from build123d import *

# Parameters (mm, degrees)
BOSS_EXTRUDE2_DEPTH = 64
CUT_EXTRUDE3_START  = -45
CUT_EXTRUDE3_DEPTH  = 45
SKETCH7_R           = 11
CUT_EXTRUDE5_DEPTH  = 96
SKETCH8_R           = 11
CUT_EXTRUDE6_DEPTH  = 105
CUT_EXTRUDE7_START  = -45
CUT_EXTRUDE7_DEPTH  = 45
SKETCH10_W          = 13
SKETCH10_H          = 64
CUT_EXTRUDE8_DEPTH  = 45
SKETCH11_W          = 13
SKETCH11_H          = 64
CUT_EXTRUDE9_DEPTH  = 45
CUT_EXTRUDE12_DEPTH = 31
CUT_EXTRUDE13_DEPTH = 31


with BuildPart() as part:
    # Sketch1 → Boss-Extrude2 (new body)
    with BuildSketch(Plane(origin=(0, 0, 0), x_dir=(1, 0, 0), z_dir=(0, 1, 0))):
        with BuildLine():
            Line((0, -32), (114, -32))
            ThreePointArc((114, -32), (146, 0), (114, 32))
            Line((114, 32), (0, 32))
            ThreePointArc((0, 32), (-32, 0), (0, -32))
        make_face()
    extrude(amount=BOSS_EXTRUDE2_DEPTH)

    # Sketch6 → Cut-Extrude3 (cut)
    with BuildSketch(Plane(origin=(0, 64, 0), x_dir=(1, 0, 0), z_dir=(0, 1, 0)).offset(CUT_EXTRUDE3_START)):
        with BuildLine():
            Line((0, 32), (0, -32))
            ThreePointArc((0, -32), (-32, 0), (0, 32))
        make_face()
    extrude(amount=CUT_EXTRUDE3_DEPTH, mode=Mode.SUBTRACT)

    # Sketch7 → Cut-Extrude5 (cut)
    with BuildSketch(Plane(origin=(0, 64, 0), x_dir=(1, 0, 0), z_dir=(0, 1, 0))):
        with Locations(Location((0, 0, 0), (0, 0, 270))):
            Circle(SKETCH7_R)
    extrude(amount=-CUT_EXTRUDE5_DEPTH, mode=Mode.SUBTRACT)

    # Sketch8 → Cut-Extrude6 (cut)
    with BuildSketch(Plane(origin=(0, 64, 0), x_dir=(1, 0, 0), z_dir=(0, 1, 0))):
        with Locations(Location((114, 0, 0), (0, 0, 270))):
            Circle(SKETCH8_R)
    extrude(amount=-CUT_EXTRUDE6_DEPTH, mode=Mode.SUBTRACT)

    # Sketch9 → Cut-Extrude7 (cut)
    with BuildSketch(Plane(origin=(0, 64, 0), x_dir=(1, 0, 0), z_dir=(0, 1, 0)).offset(CUT_EXTRUDE7_START)):
        with BuildLine():
            Line((114, 32), (114, -32))
            ThreePointArc((114, -32), (146, 0), (114, 32))
        make_face()
    extrude(amount=CUT_EXTRUDE7_DEPTH, mode=Mode.SUBTRACT)

    # Sketch10 → Cut-Extrude8 (cut)
    with BuildSketch(Plane(origin=(0, 64, 0), x_dir=(1, 0, 0), z_dir=(0, 1, 0))):
        with Locations((6.5, 0)):
            Rectangle(SKETCH10_W, SKETCH10_H)
    extrude(amount=-CUT_EXTRUDE8_DEPTH, mode=Mode.SUBTRACT)

    # Sketch11 → Cut-Extrude9 (cut)
    with BuildSketch(Plane(origin=(0, 64, 0), x_dir=(1, 0, 0), z_dir=(0, 1, 0))):
        with Locations((107.5, 0)):
            Rectangle(SKETCH11_W, SKETCH11_H)
    extrude(amount=-CUT_EXTRUDE9_DEPTH, mode=Mode.SUBTRACT)

    # Sketch15 → Cut-Extrude12 (cut)
    with BuildSketch(Plane.ZY.offset(-57)):
        Polygon((-19, 64), (32, 19), (32, 64), align=None)
    extrude(amount=-CUT_EXTRUDE12_DEPTH, mode=Mode.SUBTRACT)

    # Sketch16 → Cut-Extrude13 (cut)
    with BuildSketch(Plane(origin=(57, 0, 0), x_dir=(0, 0, -1), z_dir=(1, 0, 0))):
        Polygon((-32, 64), (19, 64), (-32, 19), align=None)
    extrude(amount=-CUT_EXTRUDE13_DEPTH, mode=Mode.SUBTRACT)


solid = part.part
Can you work these out from the model? Positions are in its coordinate system, mm. A direction names the side the tool comes from. Give positions to 0.01 mm unless a question says otherwise; leave off trailing zeros. Loops run counter-clockwise (first coordinate to the right, second up) from the corner with the lowest first, then second, coordinate; pieces in that order, holes last. Notation, with made-up numbers: (30, -0.5) -> (38, -0.5) arc R33 ccw to (38, 38.5) -> close; hole circle Ø8 at (-22, -7.5). An arc over 180 degrees is marked (long way). Write item = value, one per line.
1) For faces 4 (the flat face through (13, 42, 0)), 5 (the flat face through (56.566, 41.815, 6.143)), 6 (the flat face through (101, 42, 0)), which set-ups out of +Z, -Z, +X, -X, +Y, -Y let a thin tool reach every point of the face, with its end or its side?
Check result:
face_4 = +Z, -Z, -X, +Y
face_5 = +Z, +Y
face_6 = +Z, -Z, +X, +Y
2) Suppose I cut it at B-B on z = 2. Write out the boundary of the cut face in (x, y).
Check result:
outline = (-31.94, 0) -> (-10.82, 0) -> (-10.82, 19) -> (-31.94, 19) -> close; (10.82, 0) -> (103.18, 0) -> (103.18, 19) -> (101, 19) -> (101, 64) -> (88, 64) -> (88, 45.47) -> (26, 45.47) -> (26, 64) -> (13, 64) -> (13, 19) -> (10.82, 19) -> close; (124.82, 0) -> (145.94, 0) -> (145.94, 19) -> (124.82, 19) -> close
3) Will these pins go through, and if not, where does the flat tip stop? pin 1 (13.5 mm diameter, centred on y = 46, z = -10.5, fed in from +X); pin 2 (8 mm diameter, centred on y = 15.5, z = 20.5, fed in from +X); pin 3 (22.5 mm diameter, centred on y = 39.5, z = 7.5, fed in from -X); pin 4 (20 mm diameter, centred on x = 114, z = 0, fed in from +Y).
Check result:
pin_1 = 101
pin_2 = 141.42
pin_3 = 13
pin_4 = through
4) Suppose I cut it at C-C on x = -6.5. Write out the boundary of the cut face in (y, z), then the cut area to 3 significant figures.
Check result:
outline = (0, -31.33) -> (19, -31.33) -> (19, -8.87) -> (0, -8.87) -> close; (0, 8.87) -> (19, 8.87) -> (19, 31.33) -> (0, 31.33) -> close
area = 853 mm2
5) Suppose I cut it at D-D on y = 38.5. Write out the boundary of the cut face in (x, z), then the cut area to 3 significant figures.
Check result:
outline = (13, -32) -> (101, -32) -> (101, 32) -> (88, 32) -> (88, 9.9) -> (26, 9.9) -> (26, 32) -> (13, 32) -> close
area = 4,260 mm2
6) Thinking about a two-plate mould opening in Z: for faces 1 (the flat face through (123, 19, 7)), 2 (the cylindrical face through (124.906, 9.633, -1.432)), 3 (the cylindrical face through (145.992, 9.367, 0.704)), which applies, released by +Z, released by -Z, zero draft, split by the parting line, or undercut?
Check result:
face_1 = zero draft
face_2 = undercut
face_3 = split by the parting line
7) I need wall thicknesses on L1, parallel to X at y = 4, z = 0; L2, parallel to Z at x = 114, y = 5.75; L3, parallel to X at y = 21.5, z = 24. Which ranges of each line are inside material? Lowest first, please. Write a range as from..to.
Check result:
L1 = -32..-11, 11..103, 125..146
L2 = -32..-11, 11..32
L3 = 13..101
8) Suppose I cut it at A-A on y = 6.5. Write out the boundary of the cut face in (x, z), then the cut area to 3 significant figures.
Check result:
outline = (0, -32) -> (114, -32) arc R32 ccw to (114, 32) -> (0, 32) arc R32 ccw to start; hole circle Ø22 at (0, 0); hole circle Ø22 at (114, 0)
area = 9,750 mm2
